```python
from build123d import *

# Parameters (mm, degrees)
SKETCH1_R           = 20
BOSS_EXTRUDE1_DEPTH = 7.5
FILLET2_R           = 5
SKETCH2_R           = 3
BOSS_EXTRUDE2_DEPTH = 2
SKETCH3_R           = 1
CUT_EXTRUDE1_DEPTH  = 35.073450133


with BuildPart() as part:
    # Sketch1 → Boss-Extrude1 (new, symmetric)
    with BuildSketch(Plane.XY):
        Circle(SKETCH1_R)
    extrude(amount=BOSS_EXTRUDE1_DEPTH, both=True)

    # Fillet2
    fillet2_edges = [part.edges().sort_by_distance(p)[0] for p in [
        (-20, 0, -7.5),
        (-20, 0, 7.5),
    ]]
    fillet(fillet2_edges, radius=FILLET2_R)

    # Sketch2 → Boss-Extrude2 (add)
    with BuildSketch(Plane.XY.offset(7.5)):
        Circle(SKETCH2_R)
    boss_extrude2 = extrude(amount=BOSS_EXTRUDE2_DEPTH)

    # Mirror3: Boss-Extrude2 across plane
    add(boss_extrude2.mirror(Plane.XY))

    # Sketch3 → Cut-Extrude1 (cut, through all)
    with BuildSketch(Plane.XY.offset(9.5)):
        Circle(SKETCH3_R)
    extrude(amount=-CUT_EXTRUDE1_DEPTH, mode=Mode.SUBTRACT)


solid = part.part
```
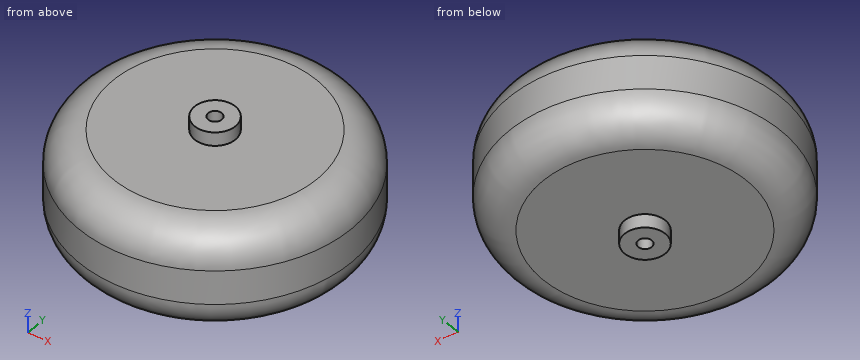
CAD build for the part. Positions are in the model's coordinates, mm. Coordinates: 2 decimals unless noted, no trailing zeros. Loops run counter-clockwise (first coordinate to the right, second up) from the corner with the lowest first, then second, coordinate; pieces in that order, holes last. Notation, with made-up numbers: (3, -32.5) - (20, -32.5) arc R7 cw to (20, -28.5) - close; hole circle Ø2 at (-13, -8). An arc over 180 degrees is marked (long way). Return JSON: item names as keys, results as strings.
1. Band-saw the part on D-D (z = -3). Give the cut face in (x, y), and give its area (3 significant figures).
Result:
{"outline": "circle Ø39.95 at (0, 0); hole circle Ø2 at (0, 0)", "area": "1,250 mm2"}
2. Drop flat-ended pins along their axis: pin 1 (1.5 mm diameter, centred on x = -4, y = 11.5, fed in from +Z); pin 2 (8 mm diameter, centred on x = 15, z = 6.5, fed in from +Y); pin 3 (1 mm diameter, centred on x = 11.5, z = 4, fed in from -Y). Give the stop position or say it passes through.
Result:
{"pin 1": "stops at z = 7.5", "pin 2": "stops at y = 15.84", "pin 3": "stops at y = -16.47"}
3. Band-saw the part on C-C (z = -5.5). Give the cut face in (x, y), and give its area (3 significant figures).
Result:
{"outline": "circle Ø38 at (0, 0); hole circle Ø2 at (0, 0)", "area": "1,130 mm2"}
4. Band-saw the part on A-A (y = 0). Give the cut face in (x, z).
Result:
{"outline": "(-20, -2.5) arc R5 ccw to (-15, -7.5) - (-3, -7.5) - (-3, -9.5) - (-1, -9.5) - (-1, 9.5) - (-3, 9.5) - (-3, 7.5) - (-15, 7.5) arc R5 ccw to (-20, 2.5) - close; (1, -9.5) - (3, -9.5) - (3, -7.5) - (15, -7.5) arc R5 ccw to (20, -2.5) - (20, 2.5) arc R5 ccw to (15, 7.5) - (3, 7.5) - (3, 9.5) - (1, 9.5) - close"}
5. Probe L1, parallel to Y at x = 0, z = -0.25; L2, parallel to Z at x = -4, y = -13; L3, parallel to Y at x = 0, z = -3.5. List the from-to ranges inside material, lowest first. Write a range as from..to.
Result:
{"L1": "y = -20..-1, 1..20", "L2": "z = -7.5..7.5", "L3": "y = -19.9..-1, 1..19.9"}
